Source: three-view drawing plus pictorial views. Frame: mm from the lowest corner of the part. Give positions to 0.01 mm unless a question says otherwise; leave off trailing zeros. Loops run counter-clockwise (first coordinate to the right, second up) from the corner with the lowest first, then second, coordinate; pieces in that order, holes last.
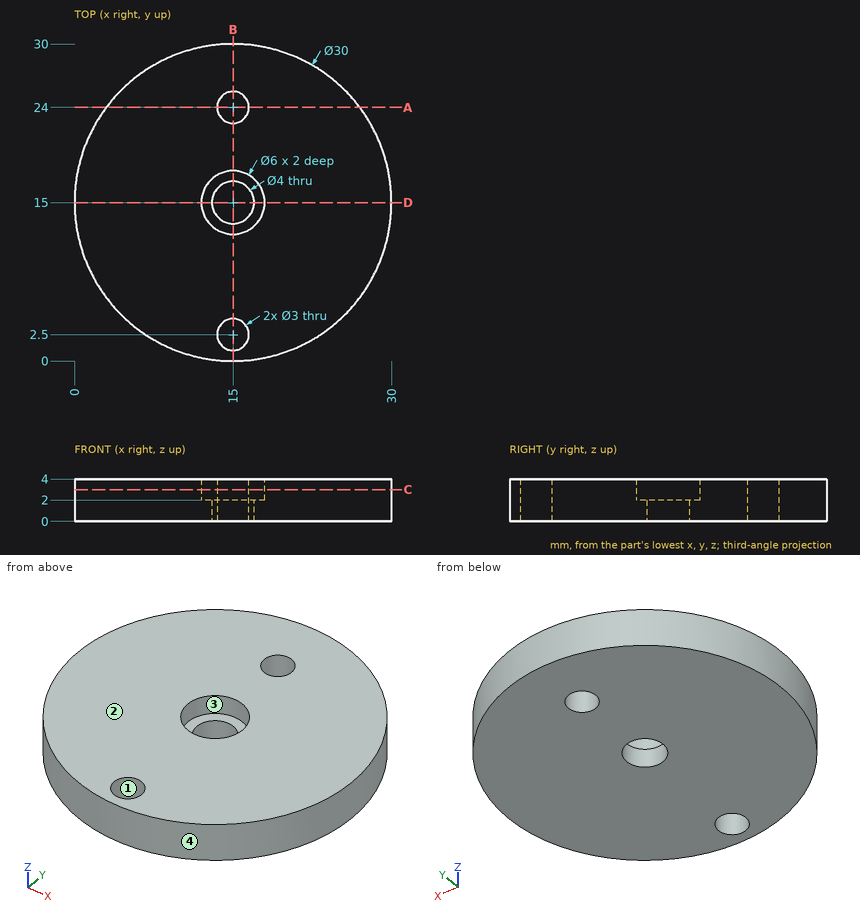
(1) Cut plane D-D (y = 15). Return the cut outline in (x, z), and give its area (3 significant figures).
Values follow:
outline: (0, 0) - (13, 0) - (13, 2) - (12, 2) - (12, 4) - (0, 4) - close; (17, 0) - (30, 0) - (30, 4) - (18, 4) - (18, 2) - (17, 2) - close
area: 100 mm2
(2) Cut plane A-A (y = 24). Return the cut outline in (x, z).
Values follow:
outline: (3, 0) - (13.5, 0) - (13.5, 4) - (3, 4) - close; (16.5, 0) - (27, 0) - (27, 4) - (16.5, 4) - close
(3) Pin query (flat end, axial travel): pin 1 Ø1 at (y, z) = (18, 1.5) entering from -X; pin 2 Ø1.5 at (x, z) = (19.5, 0.5) entering from -Y; pin 3 Ø1 at (y, z) = (5, 0.5) entering from -X. Return the tip coordinate at first contact, or that it passes through.
Values follow:
pin 1: stops at x = 0.21
pin 2: stops at y = 0.48
pin 3: stops at x = 3.39
(4) Cut plane C-C (z = 3). Return the cut outline in (x, y), and give its area (3 significant figures).
Values follow:
outline: circle Ø30 at (15, 15); hole circle Ø6 at (15, 15); hole circle Ø3 at (15, 2.5); hole circle Ø3 at (15, 24)
area: 664 mm2
(5) Mould query, pull axis X, two halves, no side actions, for the marked faces 1, 2, 3 and 4. Classes: +X half, -X half, draft (parallel to the pull), parting line (faces both ways), or undercut.
Values follow:
face 1: undercut
face 2: draft
face 3: undercut
face 4: parting line
(6) Cut plane B-B (x = 15). Return the cut outline in (y, z), and give its area (3 significant figures).
Values follow:
outline: (0, 0) - (1, 0) - (1, 4) - (0, 4) - close; (4, 0) - (13, 0) - (13, 2) - (12, 2) - (12, 4) - (4, 4) - close; (17, 0) - (22.5, 0) - (22.5, 4) - (18, 4) - (18, 2) - (17, 2) - close; (25.5, 0) - (30, 0) - (30, 4) - (25.5, 4) - close
area: 76.0 mm2
(7) Ray query, probe 1 along Y at (x, z) = (15, 0.9); probe 2 along Y at (x, z) = (15, 2.3); probe 3 along X at (y, z) = (14.5, 3.7). Return the intervals inside material, ascending.
Values follow:
probe 1: y = 0 to 1, 4 to 13, 17 to 22.5, 25.5 to 30
probe 2: y = 0 to 1, 4 to 12, 18 to 22.5, 25.5 to 30
probe 3: x = 0.01 to 12.04, 17.96 to 29.99
